Part model, mm, in its own coordinate system. Face numbers are marked on the shaded views. A direction names the side the tool comes from. Round coordinates to 2 decimals unless told otherwise and drop trailing zeros. Write each loop counter-clockwise with the first axis right and the second up, starting at its lowest first coordinate (ties: lowest second). Pieces come first, ordered by that corner, then holes. Notation, with made-up numbers: M 74,-12 L 115,-12 A29 ccw 115,25 Z; hole C 53.5,66 d1. An arc over 180 degrees is marked long. Answer as a JSON object with one key per item and string values. Group by question number.
1. Band-saw the part on C-C, the plane y = -3. Write the cut outline in (x, z).
2. Which spindle directions (+Z, -Z, +X, -X, +Y, -Y) get a long thin tool onto all of the face, cutting with end or side? Do the marked faces 1, 2 and 3. Say none if no direction does.
3. Band-saw the part on B-B, the plane z = -4.75. Write the cut outline in (x, y).
4. Drop flat-ended pins along their axis: pin 1 (1.5 mm diameter, centred on x = -13, z = 2, fed in from -Y); pin 2 (6 mm diameter, centred on x = 9, z = 3, fed in from +Y); pin 3 (6 mm diameter, centred on y = -11.5, z = 2.5, fed in from +X). Give the stop position or say it passes through.
5. Two-plate mould, pull along Y, no slides. Class the marked faces 4, 5 and 6: +Y half, -Y half, draft (parallel to the pull), parting line (faces both ways), or undercut.
6. Band-saw the part on D-D, the plane x = -12.5. Write the cut outline in (y, z).
7. Band-saw the part on A-A, the plane x = 13.5. Write the cut outline in (y, z).
8. Drill centre lines: line 1 (Y direction, x = 13, z = 4); line 2 (X direction, y = -2.5, z = -3.75); line 3 (Y direction, x = -14, z = -1.5). Where is each one in solid material? Low to high. Write a range as from..to.
from build123d import *

# Parameters (mm, degrees)
SKETCH_2_W          = 22.5
SKETCH_2_H          = 12
EXTRUDE_1_DEPTH     = 22.5
SKETCH_3_R          = 2.75
SKETCH_3_R_2        = 6
EXTRUDE_2_DEPTH     = 4.5
SKETCH_4_R          = 2.5
EXTRUDE_3_DEPTH     = 3
SKETCH_5_R          = 0.6
CUT_EXTRUDE_1_DEPTH = 3
EXTRUDE_4_DEPTH     = 2.5
FILLET_1_R          = 0.15
EXTRUDE_5_DEPTH     = 5


with BuildPart() as part:
    # ｽｹｯﾁ2 → ﾎﾞｽ - 押し出し1 (new body)
    with BuildSketch(Plane(origin=(0, 0, 0), x_dir=(1, 0, 0), z_dir=(0, 1, 0))):
        Rectangle(SKETCH_2_W, SKETCH_2_H)
    extrude(amount=-EXTRUDE_1_DEPTH)

    # ｽｹｯﾁ3 → ﾎﾞｽ - 押し出し2 (add)
    with BuildSketch(Plane(origin=(0, 0, 0), x_dir=(1, 0, 0), z_dir=(0, 1, 0))):
        Circle(SKETCH_3_R)
        with Locations((-5.25, 0)):
            Circle(SKETCH_3_R_2)
    extrude(amount=EXTRUDE_2_DEPTH)

    # ｽｹｯﾁ4 → ﾎﾞｽ - 押し出し3 (add)
    with BuildSketch(Plane(origin=(0, 4.5, 0), x_dir=(1, 0, 0), z_dir=(0, 1, 0))):
        with Locations(Location((-5.25, 0, 0), (0, 0, 270))):
            Circle(SKETCH_4_R)
    extrude(amount=EXTRUDE_3_DEPTH)

    # ｽｹｯﾁ5 → ｶｯﾄ - 押し出し1 (cut)
    with BuildSketch(Plane(origin=(0, 7.5, 0), x_dir=(1, 0, 0), z_dir=(0, 1, 0))):
        with Locations(Location((-5.25, 0, 0), (0, 0, 270))):
            Circle(SKETCH_5_R)
    extrude(amount=-CUT_EXTRUDE_1_DEPTH, mode=Mode.SUBTRACT)

    # ｽｹｯﾁ6 → ﾎﾞｽ - 押し出し4 (add)
    with BuildSketch(Plane(origin=(0, -4, 0), x_dir=(1, 0, 0), z_dir=(0, 1, 0))):
        with BuildLine():
            Line((-16.1, -0.35), (-16.1, -6))
            Line((-16.1, -6), (16.1, -6))
            Line((16.1, -6), (16.1, -0.35))
            Line((16.1, -0.35), (15.0367497, -0.35))
            ThreePointArc((15.0367497, -0.35), (13.1, 0), (15.0367497, 0.35))
            Line((15.0367497, 0.35), (16.1, 0.35))
            Line((16.1, 0.35), (16.1, 6))
            Line((16.1, 6), (-16.1, 6))
            Line((-16.1, 6), (-16.1, 0.35))
            Line((-16.1, 0.35), (-15.0367497, 0.35))
            ThreePointArc((-15.0367497, 0.35), (-13.1, 0), (-15.0367497, -0.35))
            Line((-15.0367497, -0.35), (-16.1, -0.35))
        make_face()
    extrude(amount=-EXTRUDE_4_DEPTH)

    # ﾌｨﾚｯﾄ1
    fillet_1_edges = [part.edges().sort_by_distance(p)[0] for p in [
        (16.1, -5.25, 6),
        (-16.1, -5.25, -6),
        (16.1, -5.25, -6),
        (-16.1, -5.25, 6),
    ]]
    fillet(fillet_1_edges, radius=FILLET_1_R)

    # ｽｹｯﾁ7 → ﾎﾞｽ - 押し出し5 (add)
    with BuildSketch(Plane.ZY.offset(11.25)):
        with BuildLine():
            ThreePointArc((-0.55, -18.239791576), (0, -18.6), (0.55, -18.239791576))
            ThreePointArc((0.55, -18.239791576), (1.7, -18), (0.55, -17.760208424))
            ThreePointArc((0.55, -17.760208424), (0, -17.4), (-0.55, -17.760208424))
            ThreePointArc((-0.55, -17.760208424), (-1.7, -18), (-0.55, -18.239791576))
        make_face()
    extrude(amount=EXTRUDE_5_DEPTH)


solid = part.part
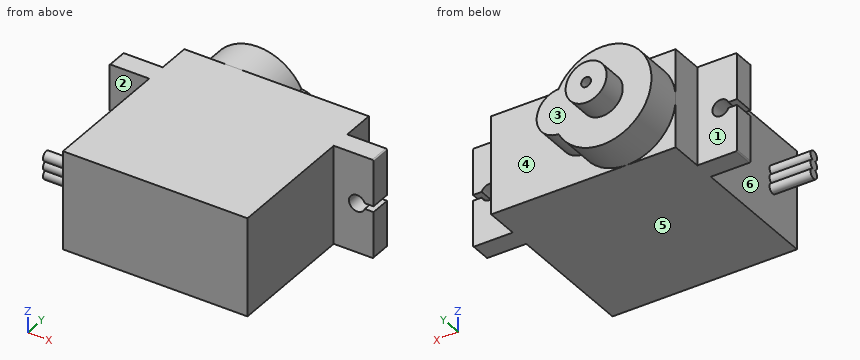
Worked answers:
{
 "1": {"outline": "M -11.25,-6 L 11.25,-6 L 11.25,6 L -11.25,6 Z"},
 "2": {"face 1": "+Z, -Z, -X, +Y", "face 2": "+Z, -Z, -X", "face 3": "+Y"},
 "3": {"outline": "M -16.1,-6.5 L -11.25,-6.5 L -11.25,-22.5 L 11.25,-22.5 L 11.25,-6.5 L 16.1,-6.5 L 16.1,-4 L 11.25,-4 L 11.25,0 L -1.58,0 L -1.58,4.5 L -8.92,4.5 L -8.92,0 L -11.25,0 L -11.25,-4 L -16.1,-4 Z"},
 "4": {"pin 1": "stops at y = -18.58", "pin 2": "stops at y = 0", "pin 3": "stops at x = 11.25"},
 "5": {"face 4": "+Y half", "face 5": "draft", "face 6": "undercut"},
 "6": {"outline": "M -18.24,-0.55 A0.6 ccw long -17.76,-0.55 A0.6 ccw -17.76,0.55 A0.6 ccw long -18.24,0.55 A0.6 ccw Z; M -6.5,-6 L -4,-6 L -4,6 L -6.5,6 Z"},
 "7": {"outline": "M -6.5,-6 L -4,-6 L -4,-0.8 L -6.5,-0.8 Z; M -6.5,0.8 L -4,0.8 L -4,6 L -6.5,6 Z"},
 "8": {"line 1": "y = -6.5..-4", "line 2": "x = -11.25..11.25", "line 3": "y = -18.45..-17.55, -6.5..-4"}
}
